Autodesk Inventor part; units mm, degrees
ref_plane "YZ Plane" through (0, 0, 0) normal (1, 0, 0) x (0, 1, 0)
ref_plane "XZ Plane" through (0, 0, 0) normal (0, 1, 0) x (-1, 0, 0)
ref_plane "XY Plane" through (0, 0, 0) normal (0, 0, 1) x (1, 0, 0)
sketch "Sketch2" plane through (0, 0, 0) normal (0, 0, 1) x (1, 0, 0)
  circle A0 centre (0, 0) radius 14.89
  circle A1 centre (0, 0) radius 9
  circle A2 centre (0, 0) radius 14.89
  line L0 (-3.6007, 8.2483) -> (-5.9571, 13.6464)
  line L1 (5.9571, 13.6464) -> (3.6007, 8.2483)
  circle A3 centre (0, 0) radius 6
  dimension "d10" = 18
  dimension "d12" = 12
extrude "Extrusion1" add sketch "Sketch2" along normal blind 10.5
extrude "Extrusion2" cut sketch "Sketch2" along normal blind 10.5 contours L1 A1 L0 A0 picked at (-1.0143, 12.8219)
pattern_circular "Circular Pattern1" count 6 over 360 about axis through (0, 0, -10) along (0, 0, 1) of "Extrusion2"
properties part number "CAO SU KHOP"
Check sheet for the modelled part. Datum: model origin and axes. Units: mm. A direction names the side the tool comes from. Round coordinates to 2 decimals unless told otherwise and drop trailing zeros. Loops run counter-clockwise (first coordinate to the right, second up) from the corner with the lowest first, then second, coordinate; pieces in that order, holes last. Notation, with made-up numbers: (-29, 63) - (25, 63) arc R22 ccw to (25, 74) - close; hole circle Ø4 at (18.5, 6). An arc over 180 degrees is marked (long way). Write item = value, one per line. Start each with the question number.
Q1. Section check A-A (y = 0). Record the boundary of the cut face in (x, z), plus the area to 3 significant figures.
Q2. Release check for a two-part mould opening along Y. For faces 4 (the face through (-7.47, 12.88, 5.18)), 5 (the face through (-7.77, -4.54, 5.18)), 6 (the face through (11.83, -1.33, 5.18)) record: pulls with the +Y half, pulls with the -Y half, needs draft (parallel to the pull), parting line crosses it, or undercut.
Q3. Section check D-D (z = 9). Record the boundary of the cut face in (x, y).
Q4. Access from +Z, -Z, +X, -X, +Y, -Y to the whole of each face (thin tool, end or side, straight path). Record for faces 1 (the face through (11.91, 1.34, 5.18)), 2 (the face through (-7.12, 9.65, 5.18)), 3 (the face through (4.762, -10.91, 5.176)).
Q5. Depth check by flat-ended pin: P1, Ø11, axis at x = 0, y = 0, coming from the +Z side; P2, Ø3, axis at x = -7.5, z = 2, coming from the +Y side; P3, Ø3, axis at y = -6.5, z = 1.5, coming from the +X side; P4, Ø6, axis at y = -6.5, z = 3.5, coming from the +X side. Enter the tip coordinate at first touch or a pass-through.
Q6. Section check C-C (x = 7.75). Record the boundary of the cut face in (y, z), plus the area to 3 significant figures.
Q7. Thickness scan on L1, parallel to Y at x = -5.5, z = 3.5; L2, parallel to X at y = 9.75, z = 4.25; L3, parallel to Y at x = 2.5, z = 3. Record the ranges inside material, lowest first.
Q8. Section check B-B (x = 0). Record the boundary of the cut face in (y, z).
Derived:
q1.outline = (-14.89, 0) - (-6, 0) - (-6, 10.5) - (-14.89, 10.5) - close; (6, 0) - (14.89, 0) - (14.89, 10.5) - (6, 10.5) - close
q1.area = 187 mm^2
q2.face_4 = pulls with the +Y half
q2.face_5 = undercut
q2.face_6 = pulls with the -Y half
q3.outline = (-14.8, -1.66) - (-8.94, -1.01) arc R9 ccw to (-5.34, -7.24) - (-8.84, -11.98) arc R14.89 ccw to (-5.96, -13.65) - (-3.6, -8.25) arc R9 ccw to (3.6, -8.25) - (5.96, -13.65) arc R14.89 ccw to (8.84, -11.98) - (5.34, -7.24) arc R9 ccw to (8.94, -1.01) - (14.8, -1.66) arc R14.89 ccw to (14.8, 1.66) - (8.94, 1.01) arc R9 ccw to (5.34, 7.24) - (8.84, 11.98) arc R14.89 ccw to (5.96, 13.65) - (3.6, 8.25) arc R9 ccw to (-3.6, 8.25) - (-5.96, 13.65) arc R14.89 ccw to (-8.84, 11.98) - (-5.34, 7.24) arc R9 ccw to (-8.94, 1.01) - (-14.8, 1.66) arc R14.89 ccw to start; hole circle Ø12 at (0, 0)
q4.face_1 = +Z, -Z, +Y
q4.face_2 = +Z, -Z, -X
q4.face_3 = +Z, -Z, -Y
q5.P1 = through
q5.P2 = 13.63
q5.P3 = 7.48
q5.P4 = 8.29
q6.outline = (-12.71, 0) - (-10.51, 0) - (-10.51, 10.5) - (-12.71, 10.5) - close; (-4.58, 0) - (4.58, 0) - (4.58, 10.5) - (-4.58, 10.5) - close; (10.51, 0) - (12.71, 0) - (12.71, 10.5) - (10.51, 10.5) - close
q6.area = 142 mm^2
q7.L1 = -12.6 to -7.46, -7.12 to -2.4, 2.4 to 7.12, 7.46 to 12.6
q7.L2 = -7.19 to -4.26, 4.26 to 7.19
q7.L3 = -8.65 to -5.45, 5.45 to 8.65
q8.outline = (-9, 0) - (-6, 0) - (-6, 10.5) - (-9, 10.5) - close; (6, 0) - (9, 0) - (9, 10.5) - (6, 10.5) - close
